Part model, mm, in its own coordinate system. Coordinates: 2 decimals unless noted, no trailing zeros. Loops run counter-clockwise (first coordinate to the right, second up) from the corner with the lowest first, then second, coordinate; pieces in that order, holes last. Notation, with made-up numbers: (-17, -12.75) - (-4, -12.75) arc R22 cw to (-4, -0.75) - close; hole circle Ø5 at (9, -23.5). An arc over 180 degrees is marked (long way). Use a Markdown table: item, result. Add a question column.
1) Band-saw the part on B-B (z = -70). Give the cut face in (x, y), plus the area to 3 significant figures.
2) Probe probe 1 along X at (y, z) = (39.5, -54); probe 2 along Y at (x, z) = (0.7, -54); probe 3 along Y at (x, z) = (4.25, -69). List the from-to ranges inside material, lowest first. Write a range as [from, to].
3) Band-saw the part on D-D (x = -6.25). Give the cut face in (y, z).
4) Band-saw the part on A-A (x = 7). Give the number of separate pieces and of enclosed holes in the cut face, plus the area to 3 significant figures.
5) Band-saw the part on C-C (z = -54). Give the cut face in (x, y), plus the area to 3 significant figures.
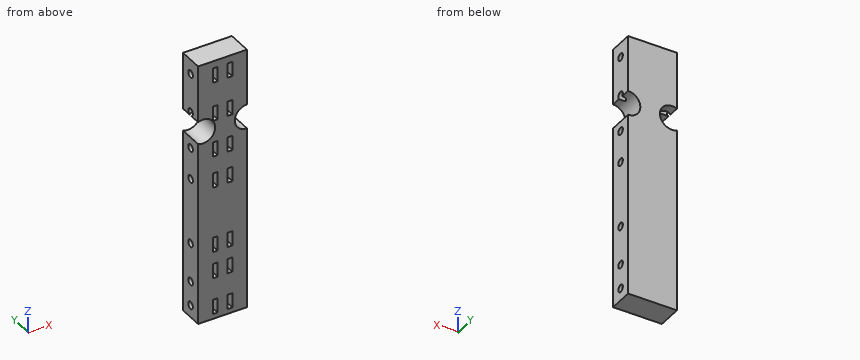
from build123d import *

# Parameters (mm, degrees)
BOX183_W               = 16
BOX183_H               = 6
BOX183_DEPTH           = 2
BOX184_W               = 16
BOX184_H               = 6
BOX184_DEPTH           = 2
BOX185_W               = 16
BOX185_H               = 6
BOX185_DEPTH           = 2
BOX186_W               = 16
BOX186_H               = 6
BOX186_DEPTH           = 2
BOX187_W               = 16
BOX187_H               = 6
BOX187_DEPTH           = 2
BOX188_W               = 16
BOX188_H               = 6
BOX188_DEPTH           = 2
BOX189_W               = 16
BOX189_H               = 6
BOX189_DEPTH           = 2
BOX190_W               = 16
BOX190_H               = 6
BOX190_DEPTH           = 2
BOX191_W               = 16
BOX191_H               = 6
BOX191_DEPTH           = 2
BOX192_W               = 16
BOX192_H               = 6
BOX192_DEPTH           = 2
BOX193_W               = 16
BOX193_H               = 6
BOX193_DEPTH           = 2
BOX194_W               = 16
BOX194_H               = 6
BOX194_DEPTH           = 2
BOX195_W               = 16
BOX195_H               = 6
BOX195_DEPTH           = 2
BOX182_W               = 16
BOX182_H               = 6
BOX182_DEPTH           = 2
CYLINDER440_R          = 1.5
CYLINDER440_DEPTH      = 50
CYLINDER441_R          = 1.5
CYLINDER441_DEPTH      = 50
CYLINDER442_R          = 1.5
CYLINDER442_DEPTH      = 50
CYLINDER443_R          = 1.5
CYLINDER443_DEPTH      = 50
CYLINDER444_R          = 1.5
CYLINDER444_DEPTH      = 50
CYLINDER445_R          = 1.5
CYLINDER445_DEPTH      = 50
CYLINDER439_R          = 1.5
CYLINDER439_DEPTH      = 50
CYLINDER432_R          = 5
CYLINDER432_DEPTH      = 100
CYLINDER433_R          = 5
CYLINDER433_DEPTH      = 100
CYLINDER434_R          = 5
CYLINDER434_DEPTH      = 100
CYLINDER435_R          = 5
CYLINDER435_DEPTH      = 100
CYLINDER436_R          = 5
CYLINDER436_DEPTH      = 100
CYLINDER437_R          = 5
CYLINDER437_DEPTH      = 100
CYLINDER438_R          = 5
CYLINDER438_DEPTH      = 100
CYLINDER431_R          = 5
CYLINDER431_DEPTH      = 100
BOX181_W               = 10
BOX181_H               = 108
BOX181_DEPTH           = 20
CUT365_ROLL_ANGLE      = 90
CUT365_PLACEMENT_ANGLE = -90


with BuildPart() as krychle183:
    # Box183 → Box183 (new body)
    with BuildSketch(Plane(origin=(60, 2, 16), x_dir=(1, 0, 0), z_dir=(0, 0, 1))):
        with Locations((8, 3)):
            Rectangle(BOX183_W, BOX183_H)
    extrude(amount=BOX183_DEPTH)


with BuildPart() as krychle184:
    # Box184 → Box184 (new body)
    with BuildSketch(Plane(origin=(60, -25, 10), x_dir=(1, 0, 0), z_dir=(0, 0, 1))):
        with Locations((8, 3)):
            Rectangle(BOX184_W, BOX184_H)
    extrude(amount=BOX184_DEPTH)


with BuildPart() as krychle185:
    # Box185 → Box185 (new body)
    with BuildSketch(Plane(origin=(60, -25, 16), x_dir=(1, 0, 0), z_dir=(0, 0, 1))):
        with Locations((8, 3)):
            Rectangle(BOX185_W, BOX185_H)
    extrude(amount=BOX185_DEPTH)


with BuildPart() as krychle186:
    # Box186 → Box186 (new body)
    with BuildSketch(Plane(origin=(60, -36, 10), x_dir=(1, 0, 0), z_dir=(0, 0, 1))):
        with Locations((8, 3)):
            Rectangle(BOX186_W, BOX186_H)
    extrude(amount=BOX186_DEPTH)


with BuildPart() as krychle187:
    # Box187 → Box187 (new body)
    with BuildSketch(Plane(origin=(60, -36, 16), x_dir=(1, 0, 0), z_dir=(0, 0, 1))):
        with Locations((8, 3)):
            Rectangle(BOX187_W, BOX187_H)
    extrude(amount=BOX187_DEPTH)


with BuildPart() as krychle188:
    # Box188 → Box188 (new body)
    with BuildSketch(Plane(origin=(60, -51, 10), x_dir=(1, 0, 0), z_dir=(0, 0, 1))):
        with Locations((8, 3)):
            Rectangle(BOX188_W, BOX188_H)
    extrude(amount=BOX188_DEPTH)


with BuildPart() as krychle189:
    # Box189 → Box189 (new body)
    with BuildSketch(Plane(origin=(60, -51, 16), x_dir=(1, 0, 0), z_dir=(0, 0, 1))):
        with Locations((8, 3)):
            Rectangle(BOX189_W, BOX189_H)
    extrude(amount=BOX189_DEPTH)


with BuildPart() as krychle190:
    # Box190 → Box190 (new body)
    with BuildSketch(Plane(origin=(60, 15, 10), x_dir=(1, 0, 0), z_dir=(0, 0, 1))):
        with Locations((8, 3)):
            Rectangle(BOX190_W, BOX190_H)
    extrude(amount=BOX190_DEPTH)


with BuildPart() as krychle191:
    # Box191 → Box191 (new body)
    with BuildSketch(Plane(origin=(60, 30, 10), x_dir=(1, 0, 0), z_dir=(0, 0, 1))):
        with Locations((8, 3)):
            Rectangle(BOX191_W, BOX191_H)
    extrude(amount=BOX191_DEPTH)


with BuildPart() as krychle192:
    # Box192 → Box192 (new body)
    with BuildSketch(Plane(origin=(60, 46, 10), x_dir=(1, 0, 0), z_dir=(0, 0, 1))):
        with Locations((8, 3)):
            Rectangle(BOX192_W, BOX192_H)
    extrude(amount=BOX192_DEPTH)


with BuildPart() as krychle193:
    # Box193 → Box193 (new body)
    with BuildSketch(Plane(origin=(60, 15, 16), x_dir=(1, 0, 0), z_dir=(0, 0, 1))):
        with Locations((8, 3)):
            Rectangle(BOX193_W, BOX193_H)
    extrude(amount=BOX193_DEPTH)


with BuildPart() as krychle194:
    # Box194 → Box194 (new body)
    with BuildSketch(Plane(origin=(60, 30, 16), x_dir=(1, 0, 0), z_dir=(0, 0, 1))):
        with Locations((8, 3)):
            Rectangle(BOX194_W, BOX194_H)
    extrude(amount=BOX194_DEPTH)


with BuildPart() as krychle195:
    # Box195 → Box195 (new body)
    with BuildSketch(Plane(origin=(60, 46, 16), x_dir=(1, 0, 0), z_dir=(0, 0, 1))):
        with Locations((8, 3)):
            Rectangle(BOX195_W, BOX195_H)
    extrude(amount=BOX195_DEPTH)


with BuildPart() as compound585:
    # Box182 → Box182 (new body)
    with BuildSketch(Plane(origin=(60, 2, 10), x_dir=(1, 0, 0), z_dir=(0, 0, 1))):
        with Locations((8, 3)):
            Rectangle(BOX182_W, BOX182_H)
    extrude(amount=BOX182_DEPTH)

    # Compound585: union Krychle183, Krychle184, Krychle185, Krychle186, Krychle187, Krychle188, Krychle189, Krychle190, Krychle191, Krychle192, Krychle193, Krychle194, Krychle195
    add(krychle183.part)
    add(krychle184.part)
    add(krychle185.part)
    add(krychle186.part)
    add(krychle187.part)
    add(krychle188.part)
    add(krychle189.part)
    add(krychle190.part)
    add(krychle191.part)
    add(krychle192.part)
    add(krychle193.part)
    add(krychle194.part)
    add(krychle195.part)


with BuildPart() as compound585_1:
    # Compound585 placement: moved
    add(compound585.part.moved(Location((39, 24, 3))))


with BuildPart() as obj1:
    # Cylinder440 → Cylinder440 (new body)
    with BuildSketch(Plane(origin=(63, -22, -12), x_dir=(1, 0, 0), z_dir=(0, 0, 1))):
        Circle(CYLINDER440_R)
    extrude(amount=CYLINDER440_DEPTH)


with BuildPart() as obj2:
    # Cylinder441 → Cylinder441 (new body)
    with BuildSketch(Plane(origin=(63, -38, -12), x_dir=(1, 0, 0), z_dir=(0, 0, 1))):
        Circle(CYLINDER441_R)
    extrude(amount=CYLINDER441_DEPTH)


with BuildPart() as obj3:
    # Cylinder442 → Cylinder442 (new body)
    with BuildSketch(Plane(origin=(63, -48, -12), x_dir=(1, 0, 0), z_dir=(0, 0, 1))):
        Circle(CYLINDER442_R)
    extrude(amount=CYLINDER442_DEPTH)


with BuildPart() as obj4:
    # Cylinder443 → Cylinder443 (new body)
    with BuildSketch(Plane(origin=(63, 18, -12), x_dir=(1, 0, 0), z_dir=(0, 0, 1))):
        Circle(CYLINDER443_R)
    extrude(amount=CYLINDER443_DEPTH)


with BuildPart() as obj5:
    # Cylinder444 → Cylinder444 (new body)
    with BuildSketch(Plane(origin=(63, 33, -12), x_dir=(1, 0, 0), z_dir=(0, 0, 1))):
        Circle(CYLINDER444_R)
    extrude(amount=CYLINDER444_DEPTH)


with BuildPart() as obj6:
    # Cylinder445 → Cylinder445 (new body)
    with BuildSketch(Plane(origin=(63, 49, -12), x_dir=(1, 0, 0), z_dir=(0, 0, 1))):
        Circle(CYLINDER445_R)
    extrude(amount=CYLINDER445_DEPTH)


with BuildPart() as compound590:
    # Cylinder439 → Cylinder439 (new body)
    with BuildSketch(Plane(origin=(63, 5, -12), x_dir=(1, 0, 0), z_dir=(0, 0, 1))):
        Circle(CYLINDER439_R)
    extrude(amount=CYLINDER439_DEPTH)

    # Compound590: union obj1, obj2, obj3, obj4, obj5, obj6
    add(obj1.part)
    add(obj2.part)
    add(obj3.part)
    add(obj4.part)
    add(obj5.part)
    add(obj6.part)


with BuildPart() as compound590_1:
    # Compound590 placement: moved
    add(compound590.part.moved(Location((39, 24, 0))))


with BuildPart() as obj7:
    # Cylinder432 → Cylinder432 (new body)
    with BuildSketch(Plane(origin=(24, -51, 25), x_dir=(0, 0, -1), z_dir=(1, 0, 0))):
        Circle(CYLINDER432_R)
    extrude(amount=CYLINDER432_DEPTH)


with BuildPart() as obj8:
    # Cylinder433 → Cylinder433 (new body)
    with BuildSketch(Plane(origin=(24, 36, 34), x_dir=(0, 0, -1), z_dir=(1, 0, 0))):
        Circle(CYLINDER433_R)
    extrude(amount=CYLINDER433_DEPTH)


with BuildPart() as obj9:
    # Cylinder434 → Cylinder434 (new body)
    with BuildSketch(Plane(origin=(24, -36, 34), x_dir=(0, 0, -1), z_dir=(1, 0, 0))):
        Circle(CYLINDER434_R)
    extrude(amount=CYLINDER434_DEPTH)


with BuildPart() as obj10:
    # Cylinder435 → Cylinder435 (new body)
    with BuildSketch(Plane(origin=(24, -23, -5), x_dir=(0, 0, -1), z_dir=(1, 0, 0))):
        Circle(CYLINDER435_R)
    extrude(amount=CYLINDER435_DEPTH)


with BuildPart() as obj11:
    # Cylinder436 → Cylinder436 (new body)
    with BuildSketch(Plane(origin=(24, 51, 7), x_dir=(0, 0, -1), z_dir=(1, 0, 0))):
        Circle(CYLINDER436_R)
    extrude(amount=CYLINDER436_DEPTH)


with BuildPart() as obj12:
    # Cylinder437 → Cylinder437 (new body)
    with BuildSketch(Plane(origin=(24, 23, -5), x_dir=(0, 0, -1), z_dir=(1, 0, 0))):
        Circle(CYLINDER437_R)
    extrude(amount=CYLINDER437_DEPTH)


with BuildPart() as obj13:
    # Cylinder438 → Cylinder438 (new body)
    with BuildSketch(Plane(origin=(24, -51, 7), x_dir=(0, 0, -1), z_dir=(1, 0, 0))):
        Circle(CYLINDER438_R)
    extrude(amount=CYLINDER438_DEPTH)


with BuildPart() as compound589:
    # Cylinder431 → Cylinder431 (new body)
    with BuildSketch(Plane(origin=(24, 51, 25), x_dir=(0, 0, -1), z_dir=(1, 0, 0))):
        Circle(CYLINDER431_R)
    extrude(amount=CYLINDER431_DEPTH)

    # Compound589: union obj7, obj8, obj9, obj10, obj11, obj12, obj13
    add(obj7.part)
    add(obj8.part)
    add(obj9.part)
    add(obj10.part)
    add(obj11.part)
    add(obj12.part)
    add(obj13.part)


with BuildPart() as compound589_1:
    # Compound589 placement: moved
    add(compound589.part.moved(Location((32, 0, 0))))


with BuildPart() as obj14:
    # Box181 → Box181 (new body)
    with BuildSketch(Plane(origin=(97, -29, 7), x_dir=(1, 0, 0), z_dir=(0, 0, 1))):
        with Locations((5, 54)):
            Rectangle(BOX181_W, BOX181_H)
    extrude(amount=BOX181_DEPTH)

    # Cut363: cut Compound589
    add(compound589_1.part, mode=Mode.SUBTRACT)

    # Cut364: cut Compound590
    add(compound590_1.part, mode=Mode.SUBTRACT)

    # Cut365: cut Compound585
    add(compound585_1.part, mode=Mode.SUBTRACT)


with BuildPart() as obj14_1:
    # Cut365 roll: moved
    add(obj14.part.rotate(Axis((0, 0, 0), (1, 0, 0)), CUT365_ROLL_ANGLE))


with BuildPart() as obj14_2:
    # Cut365 placement: moved
    add(obj14_1.part.moved(Location((17, 144, -56))).rotate(Axis((17, 144, -56), (0, 0, 1)), CUT365_PLACEMENT_ANGLE))


solid = obj14_2.part
Answer block:
| question | item | result |
|---|---|---|
| 1 | outline | (-10, 37) - (10, 37) - (10, 40.5) - (-10, 40.5) - close; (-10, 43.5) - (10, 43.5) - (10, 47) - (-10, 47) - close |
| 1 | area | 140 mm2 |
| 2 | probe 1 | [-10, -4], [-2, 2], [4, 10] |
| 2 | probe 2 | [37, 40.5], [43.5, 47] |
| 2 | probe 3 | [37, 40.88], [43.12, 47] |
| 3 | outline | (37, -85) - (47, -85) - (47, -9.68) - (37, -9.68) - close; (37, -0.32) - (41.28, -0.32) arc R1.5 cw (long way) to (42.72, -0.32) - (47, -0.32) - (47, 23) - (37, 23) - close; hole circle Ø3 at (42, -80); hole circle Ø3 at (42, -70); hole circle Ø3 at (42, -54); hole circle Ø3 at (42, -27); hole circle Ø3 at (42, -14); hole circle Ø3 at (42, 17) |
| 4 | separate pieces | 2 |
| 4 | enclosed holes | 7 |
| 4 | area | 951 mm2 |
| 5 | outline | (-10, 37) - (-4, 37) - (-4, 40.5) - (-10, 40.5) - close; (-10, 43.5) - (-4, 43.5) - (-4, 45) - (-2, 45) - (-2, 43.5) - (2, 43.5) - (2, 45) - (4, 45) - (4, 43.5) - (10, 43.5) - (10, 47) - (-10, 47) - close; (-2, 37) - (2, 37) - (2, 40.5) - (-2, 40.5) - close; (4, 37) - (10, 37) - (10, 40.5) - (4, 40.5) - close |
| 5 | area | 120 mm2 |
